Source: three-view drawing plus pictorial views. Frame: mm from the lowest corner of the part. Coordinates: 2 decimals unless noted, no trailing zeros. Order: outer loops, then holes, each group sorted by start corner. A loop starts at its lowest first (then second) coordinate and runs counter-clockwise, first axis right, second up. Notation, with made-up numbers: (81, 5.25) -> (119, 5.25) arc R25 cw to (119, 38.25) -> close; hole circle Ø8 at (50.5, -19). An arc over 180 degrees is marked (long way). Use one line per item in the form item = value. Start each with the question number.
1) Ray query, line 1 along Y through (x, z) = (63, 33); line 2 along Y through (x, z) = (72.5, 72); line 3 along Z through (x, y) = (38, 13.5) (1 decimal). Return the intervals inside material, ascending.
2) Section query B-B on x = 19. Output: boundary loops of the cut face in (y, z).
3) Section query D-D on y = 8.75. Output: boundary loops of the cut face in (x, z), then the cut area to 3 significant figures.
4) Draft query along Z for the marked faces 1, 2 and 3. Return one class per face: pulls with the +Z half, pulls with the -Z half, needs draft (parallel to the pull), parting line crosses it, or undercut.
5) Section query C-C on z = 28. Output: boundary loops of the cut face in (x, y).
6) Section query A-A on y = 1.5. Output: boundary loops of the cut face in (x, z).
7) Pin query (flat end, axial travel): pin 1 (1 mm diameter, centred on y = 8.5, z = 10, fed in from -X); pin 2 (2 mm diameter, centred on x = 59.5, y = 4, fed in from +Z); pin 3 (4 mm diameter, centred on y = 9, z = 50, fed in from -X); pin 4 (4 mm diameter, centred on x = 20, y = 8, fed in from +Z). Return the tip coordinate at first contact, or that it passes through.
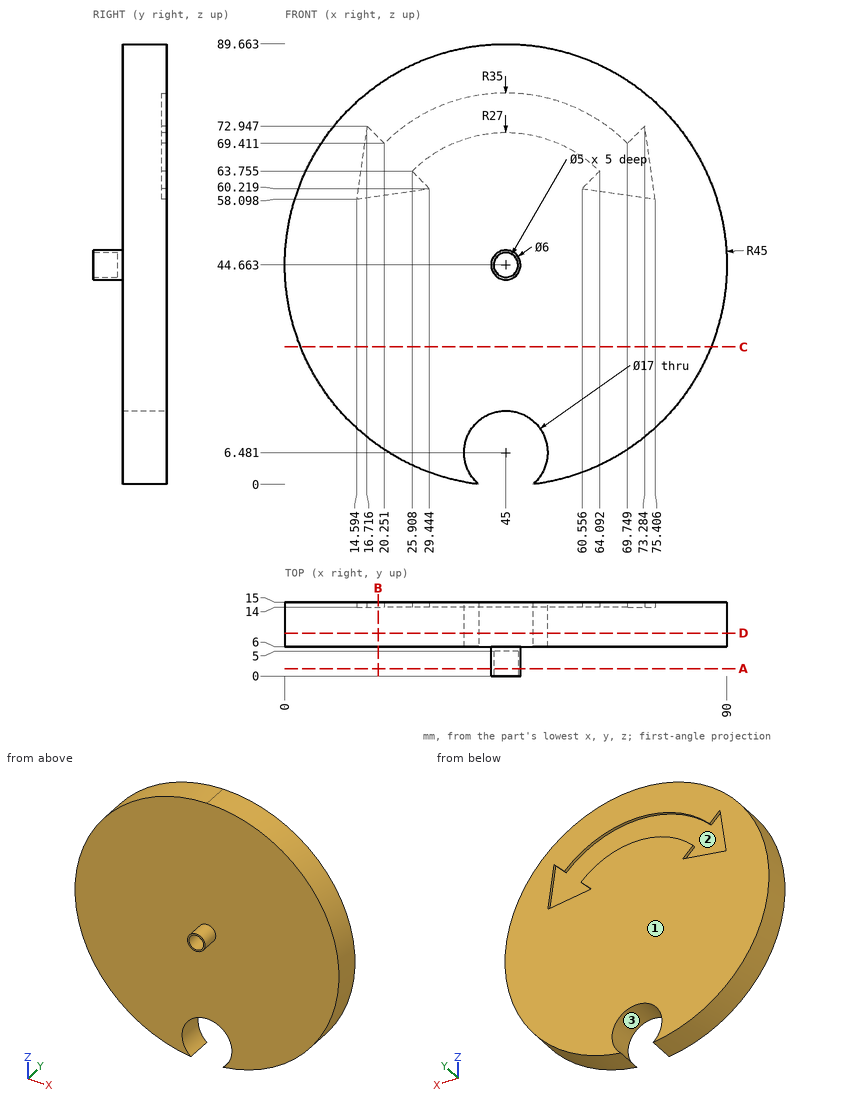
Answers below:
q1.line_1 = 6 to 15
q1.line_2 = 6 to 14
q1.line_3 = 0.2 to 1.7, 11.3 to 89.1
q2.outline = (6, 7.93) -> (15, 7.93) -> (15, 58.73) -> (14, 58.73) -> (14, 70.66) -> (15, 70.66) -> (15, 81.39) -> (6, 81.39) -> close
q3.outline = (39.5, 0) arc R8.5 cw (long way) to (50.5, 0) arc R45 ccw (long way) to start
q3.area = 6,150 mm^2
q4.face_1 = needs draft
q4.face_2 = undercut
q4.face_3 = undercut
q5.outline = (3.2, 6) -> (86.8, 6) -> (86.8, 15) -> (3.2, 15) -> close
q6.outline = circle Ø6 at (45, 44.66); hole circle Ø5 at (45, 44.66)
q7.pin_1 = 15.71
q7.pin_2 = through
q7.pin_3 = 0.12
q7.pin_4 = 83.34
